```python
from build123d import *

# Parameters (mm, degrees)
F0_W     = 18
F0_H     = 18
F1_DEPTH = 7
F2_SIZE2 = 6.99999
F2_SIZE  = 2.99999
F3_R     = 2.55
F4_DEPTH = 25


# Not quite as in the source:
# - a fillet or chamfer is up to 0.001 mm smaller than in the source, because OpenCascade refuses the exact size


with BuildPart() as f1:
    # F0 (on Top) → F1 (new body)
    with BuildSketch(Plane.XY):
        Rectangle(F0_W, F0_H)
    extrude(amount=F1_DEPTH)

    # F2 (size 3 and 7 in the source; OpenCascade refuses exactly that, so slightly less here)
    f2_edges = [f1.edges().sort_by_distance(p)[0] for p in [
        (-9, 0, 7),
        (0, 9, 7),
        (9, 0, 7),
        (0, -9, 7),
    ]]
    f2_side = f1.faces().sort_by_distance((0, 0, 7))[0]
    chamfer(f2_edges, length=F2_SIZE, length2=F2_SIZE2, reference=f2_side)

    # F3 (on Top) → F4 (cut)
    with BuildSketch(Plane.XY):
        Circle(F3_R)
    extrude(amount=F4_DEPTH, mode=Mode.SUBTRACT)


solid = f1.part
```
Input: part model. Units: mm. Frame: model coordinates. Coordinates: 2 decimals unless noted, no trailing zeros. Write each loop counter-clockwise with the first axis right and the second up, starting at its lowest first coordinate (ties: lowest second). Pieces come first, ordered by that corner, then holes.
1) Section D-D on z = 5.75. Output: boundary loops of the cut face in (x, y).
2) Pin query (flat end, axial travel): pin 1 Ø4 at (x, z) = (-4.5, 4.5) entering from +Y; pin 2 Ø3 at (x, z) = (-3, 3) entering from -Y. Return the tip coordinate at first contact, or that it passes through.
3) Mould query, pull axis Y, two halves, no side actions, for faces 1 (the flat face through (-0.1, -7.5, 3.5)), 2 (the cylindrical face through (1.18, -2.26, 3.45)), 3 (the flat face through (-0.1, 7.5, 3.5)). Classes: pulls with the +Y half, pulls with the -Y half, needs draft (parallel to the pull), parting line crosses it, or undercut.
4) Material intervals for line 1 along X through (y, z) = (-0.25, 6.25); line 2 along X through (y, z) = (0, 1.75); line 3 along Y through (x, z) = (-4, 3.75), sorted ascending.
Check result:
1. outline: (-6.54, -6.54) - (6.54, -6.54) - (6.54, 6.54) - (-6.54, 6.54) - close; hole circle Ø5.1 at (0, 0)
2. pin 1: stops at y = 7.93
2. pin 2: stops at y = -8.36
3. face 1: pulls with the -Y half
3. face 2: undercut
3. face 3: pulls with the +Y half
4. line 1: x = -6.32 to -2.54, 2.54 to 6.32
4. line 2: x = -8.25 to -2.55, 2.55 to 8.25
4. line 3: y = -7.39 to 7.39
